```python
from build123d import *

# Parameters (mm, degrees)
SKETCH1_W           = 40
SKETCH1_H           = 6
SKETCH1_R           = 2.06
BOSS_EXTRUDE1_DEPTH = 25
BOSS_EXTRUDE2_DEPTH = 10
BOSS_EXTRUDE4_START = 4
SKETCH4_W           = 5
SKETCH4_H           = 36
BOSS_EXTRUDE4_DEPTH = 4
SKETCH5_W           = 10
SKETCH5_H           = 18
CUT_EXTRUDE1_DEPTH  = 8


with BuildPart() as part:
    # Sketch1 → Boss-Extrude1 (new body)
    with BuildSketch(Plane(origin=(0, 0, 0), x_dir=(0, 1, 0), z_dir=(0, 0, 1))):
        with Locations((4.5125, -0.675)):
            Rectangle(SKETCH1_W, SKETCH1_H)
        with Locations(Location((-12.4875, -0.675, 0), (0, 0, 270))):
            Circle(SKETCH1_R, mode=Mode.SUBTRACT)
        with Locations(Location((21.5125, -0.675, 0), (0, 0, 90))):
            Circle(SKETCH1_R, mode=Mode.SUBTRACT)
    extrude(amount=BOSS_EXTRUDE1_DEPTH)

    # Sketch2 → Boss-Extrude2 (add)
    with BuildSketch(Plane(origin=(0, 0, 0), x_dir=(1, 0, 0), z_dir=(0, 0, -1))):
        Polygon((-2.325, 15.4875), (3.675, 15.4875), (3.675, 17.4875), (-32.325, 17.4875), (-32.325, 13.4875), (-2.325, 13.4875), align=None)
        Polygon((3.675, -26.5125), (3.675, -24.5125), (-2.325, -24.5125), (-2.325, -22.5125), (-32.325, -22.5125), (-32.325, -26.5125), align=None)
    extrude(amount=-BOSS_EXTRUDE2_DEPTH)

    # Sketch4 → Boss-Extrude4 (add)
    with BuildSketch(Plane(origin=(0, 0, 0), x_dir=(1, 0, 0), z_dir=(0, 0, -1)).offset(BOSS_EXTRUDE4_START)):
        with BuildLine():
            Line((3.675, 17.4875), (-32.325, 17.4875))
            Line((-32.325, 17.4875), (-32.325, 13.4875))
            Line((-32.325, 13.4875), (-27.325, 13.4875))
            Line((-27.325, 13.4875), (-14.325, 13.4875))
            Line((-14.325, 13.4875), (-9.325, 13.4875))
            Line((-9.325, 13.4875), (-2.325, 13.4875))
            Line((-2.325, 13.4875), (-1.125999722, 13.4875))
            ThreePointArc((-1.125999722, 13.4875), (0.675, 14.5475), (2.475999722, 13.4875))
            Line((2.475999722, 13.4875), (3.675, 13.4875))
            Line((3.675, 13.4875), (3.675, 17.4875))
        make_face()
        with BuildLine():
            ThreePointArc((2.735, 12.4875), (2.669199016, 13.003998099), (2.475999722, 13.4875))
            Line((2.475999722, 13.4875), (-1.125999722, 13.4875))
            ThreePointArc((-1.125999722, 13.4875), (0.158501901, 10.493300984), (2.735, 12.4875))
        make_face()
        with BuildLine():
            Line((-1.125999722, 13.4875), (2.475999722, 13.4875))
            ThreePointArc((2.475999722, 13.4875), (0.675, 14.5475), (-1.125999722, 13.4875))
        make_face()
        with BuildLine():
            Line((3.675, -22.5125), (3.675, 13.4875))
            Line((3.675, 13.4875), (2.475999722, 13.4875))
            ThreePointArc((2.475999722, 13.4875), (2.669199016, 13.003998099), (2.735, 12.4875))
            ThreePointArc((2.735, 12.4875), (0.158501901, 10.493300984), (-1.125999722, 13.4875))
            Line((-1.125999722, 13.4875), (-2.325, 13.4875))
            Line((-2.325, 13.4875), (-2.325, -22.5125))
            Line((-2.325, -22.5125), (-1.125999722, -22.5125))
            ThreePointArc((-1.125999722, -22.5125), (0.158501901, -19.518300984), (2.735, -21.5125))
            ThreePointArc((2.735, -21.5125), (2.669199016, -22.028998099), (2.475999722, -22.5125))
            Line((2.475999722, -22.5125), (3.675, -22.5125))
        make_face()
        with BuildLine():
            ThreePointArc((-1.125999722, -22.5125), (0.675, -23.5725), (2.475999722, -22.5125))
            Line((2.475999722, -22.5125), (-1.125999722, -22.5125))
        make_face()
        with BuildLine():
            Line((-1.125999722, -22.5125), (2.475999722, -22.5125))
            ThreePointArc((2.475999722, -22.5125), (2.669199016, -22.028998099), (2.735, -21.5125))
            ThreePointArc((2.735, -21.5125), (0.158501901, -19.518300984), (-1.125999722, -22.5125))
        make_face()
        with BuildLine():
            Line((-27.325, -22.5125), (-32.325, -22.5125))
            Line((-32.325, -22.5125), (-32.325, -26.5125))
            Line((-32.325, -26.5125), (3.675, -26.5125))
            Line((3.675, -26.5125), (3.675, -22.5125))
            Line((3.675, -22.5125), (2.475999722, -22.5125))
            ThreePointArc((2.475999722, -22.5125), (0.675, -23.5725), (-1.125999722, -22.5125))
            Line((-1.125999722, -22.5125), (-2.325, -22.5125))
            Line((-2.325, -22.5125), (-9.325, -22.5125))
            Line((-9.325, -22.5125), (-14.325, -22.5125))
            Line((-14.325, -22.5125), (-27.325, -22.5125))
        make_face()
        with Locations((-29.825, -4.5125)):
            Rectangle(SKETCH4_W, SKETCH4_H)
        with Locations((-11.825, -4.5125)):
            Rectangle(SKETCH4_W, SKETCH4_H)
    extrude(amount=-BOSS_EXTRUDE4_DEPTH)

    # Sketch5 → Cut-Extrude1 (cut)
    with BuildSketch(Plane(origin=(-2.325, 0, 0), x_dir=(0, -1, 0), z_dir=(-1, 0, 0))):
        with Locations((4.4875, 12)):
            Rectangle(SKETCH5_W, SKETCH5_H)
    extrude(amount=-CUT_EXTRUDE1_DEPTH, mode=Mode.SUBTRACT)


solid = part.part
```
Can you work these out from the model? Positions are in its coordinate system, mm. A direction names the side the tool comes from. Give positions to 0.01 mm unless a question says otherwise; leave off trailing zeros. Loops run counter-clockwise (first coordinate to the right, second up) from the corner with the lowest first, then second, coordinate; pieces in that order, holes last. Notation, with made-up numbers: M 83.25,76.25 L 98.25,76.25 A26 ccw 98.25,106.25 Z; hole C -19,-7 d9. An arc over 180 degrees is marked long. Use one line per item in the form item = value. Start each with the question number.
(1) On a 3-axis mill with a long thin cutter (end or side, diameter ignored), from which of +Z, -Z, +X, -X, +Y, -Y can I reach the whole of each face in a straight line? I mean faces 4 (the flat face through (1, -15.488, 17)), 5 (the flat face through (1, -4, 3)), 6 (the flat face through (-17, 22.512, 3)). Say none if no direction works.
(2) I want a section at A-A, the plane y = 5. Write out the boundary of the cut face in (x, z) (3 decimals).
(3) I want a section at B-B, the plane z = -1.25. Write out the boundary of the cut face in (x, y) (1 decimal).
(4) Thinking about a two-plate mould opening in Z: for faces 1 (the flat face through (1, 4, 25)), 2 (the flat face through (1, -9.488, 12)), 3 (the flat face through (-18, -13.488, 4)), which applies, released by +Z, released by -Z, zero draft, split by the parting line, or undercut?
(5) I want a section at C-C, the plane x = -15. Write out the boundary of the cut face in (y, z).
(6) Please list where these lines run through material, in increasing order: line 1 (X direction, y = -0.5, z = -1.25) (3 decimals); line 2 (Y direction, x = -24.5, z = 8.75); line 3 (Y direction, x = 2, z = 12).
(7) I want a section at D-D, the plane z = 4.25. Write out the boundary of the cut face in (x, y) (1 decimal).
(8) I'm going to push flat-ended pins straight in: P1, Ø3, axis at x = -27.5, y = 19, coming from the +Z side; P2, Ø3, axis at x = -23, y = -16.5, coming from the +Z side; P3, Ø5, axis at x = 1, z = 15, coming from the +Y side. Where does each tip first touch, or does it pass through?
Worked out:
q1.face_4 = +Z, +X, -X, -Y
q1.face_5 = +X, -X
q1.face_6 = +Z
q2.outline = M -32.325,-4 L -27.325,-4 L -27.325,0 L -32.325,0 Z; M -14.325,-4 L -9.325,-4 L -9.325,0 L -14.325,0 Z; M -2.325,-4 L 3.675,-4 L 3.675,25 L -2.325,25 Z
q3.outline = M -32.3,-17.5 L 3.7,-17.5 L 3.7,26.5 L -32.3,26.5 Z; hole M -27.3,-13.5 L -14.3,-13.5 L -14.3,22.5 L -27.3,22.5 Z; hole M -9.3,-13.5 L -2.3,-13.5 L -2.3,22.5 L -9.3,22.5 Z
q4.face_1 = released by +Z
q4.face_2 = undercut
q4.face_3 = zero draft
q5.outline = M -17.49,-4 L -13.49,-4 L -13.49,10 L -17.49,10 Z; M 22.51,-4 L 26.51,-4 L 26.51,10 L 22.51,10 Z
q6.line_1 = -32.325 to -27.325, -14.325 to -9.325, -2.325 to 3.675
q6.line_2 = -17.49 to -13.49, 22.51 to 26.51
q6.line_3 = -15.49 to -14.06, -10.91 to -9.49, 0.51 to 19.94, 23.09 to 24.51
q7.outline = M -32.3,-17.5 L 3.7,-17.5 L 3.7,-9.5 L -2.3,-9.5 L -2.3,-13.5 L -32.3,-13.5 Z; M -32.3,22.5 L -2.3,22.5 L -2.3,0.5 L 3.7,0.5 L 3.7,26.5 L -32.3,26.5 Z; hole C 0.7,-12.5 d4.1; hole C 0.7,21.5 d4.1
q8.P1 = 0
q8.P2 = 10
q8.P3 = 24.51
